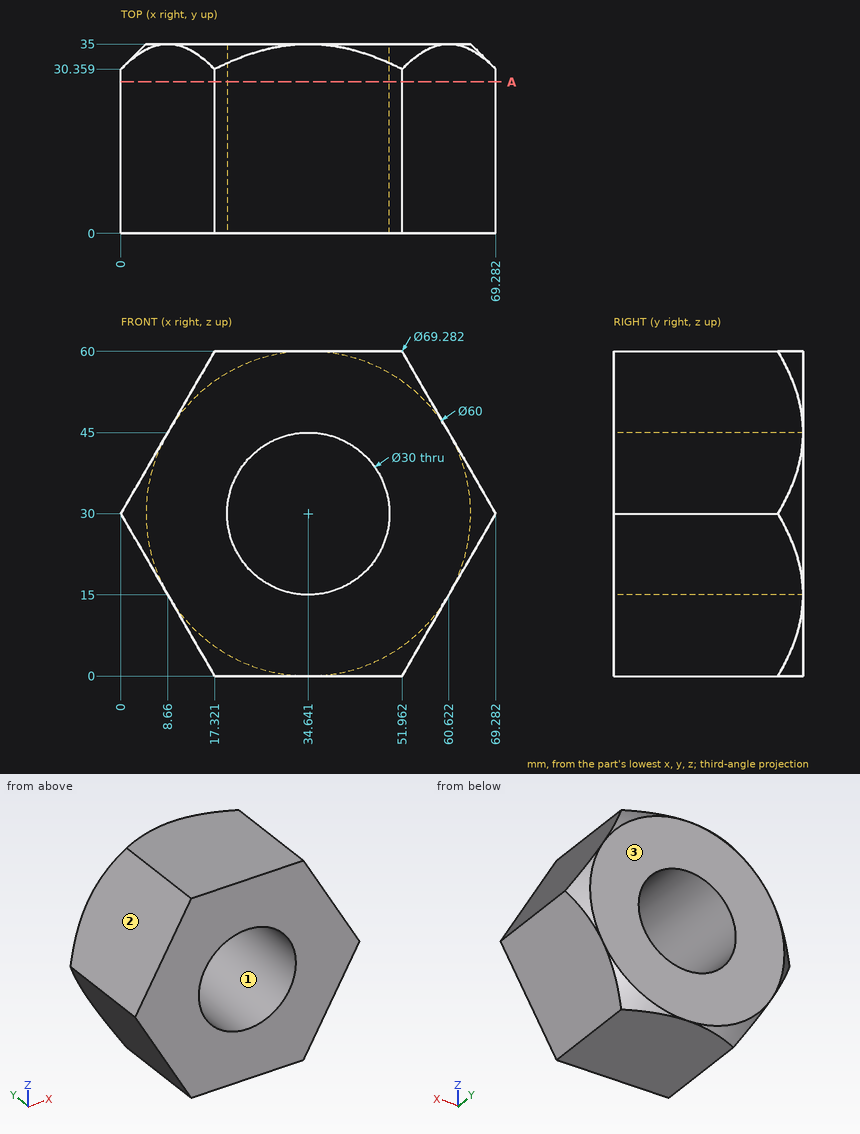
Geometry check sheet. Reference: drawing and pictorial views, mm from the part's lowest x, y, z. Coordinates: 2 decimals unless noted, no trailing zeros. Loops run counter-clockwise (first coordinate to the right, second up) from the corner with the lowest first, then second, coordinate; pieces in that order, holes last. Notation, with made-up numbers: (-24.5, 71.5) -> (-16.5, 71.5) arc R30 ccw to (-16.5, 96.5) -> close; hole circle Ø3 at (13, 37). An arc over 180 degrees is marked (long way). Write item = value, one per line. Start each with the question number.
1. Depth check by flat-ended pin: P1, Ø6, axis at x = 11.5, y = 4, coming from the +Z side (1 decimal); P2, Ø24, axis at x = 34.64, z = 30, coming from the -Y side; P3, Ø1, axis at y = 17.5, z = 27.5, coming from the -X side (1 decimal). Enter the tip coordinate at first touch or a pass-through.
2. Section check A-A on y = 28. Record the cut outline in (x, z), then the cut area to 3 significant figures.
3. Draft check along Z on the marked faces 1, 2 and 3. Enter one of: released by +Z, released by -Z, zero draft, split by the parting line, or undercut.
4. Material ranges on line 1 (Z direction, x = 39.5, y = 27); line 2 (X direction, y = 9, z = 34) (1 decimal); line 3 (X direction, y = 12.5, z = 35) (1 decimal), recorded low to high.
Responses:
q1.P1 = 55.1
q1.P2 = through
q1.P3 = 1.2
q2.outline = (0, 30) -> (17.32, 0) -> (51.96, 0) -> (69.28, 30) -> (51.96, 60) -> (17.32, 60) -> close; hole circle Ø30 at (34.64, 30)
q2.area = 2,410 mm2
q3.face_1 = undercut
q3.face_2 = released by +Z
q3.face_3 = zero draft
q4.line_1 = 0 to 15.81, 44.19 to 60
q4.line_2 = 2.3 to 20.2, 49.1 to 67
q4.line_3 = 2.9 to 20.5, 48.8 to 66.4
